```python
from build123d import *

# Parameters (mm, degrees)
SKETCH1_R           = 17.78
BOSS_EXTRUDE1_DEPTH = 1.5875
CUT_EXTRUDE1_DEPTH  = 2.5875


with BuildPart() as part:
    # Sketch1 → Boss-Extrude1 (new body)
    with BuildSketch(Plane(origin=(0, 0, 0), x_dir=(1, 0, 0), z_dir=(0, 1, 0))):
        Circle(SKETCH1_R)
    extrude(amount=BOSS_EXTRUDE1_DEPTH)

    # Sketch2 → Cut-Extrude1 (cut, through all)
    with BuildSketch(Plane(origin=(0, 1.5875, 0), x_dir=(1, 0, 0), z_dir=(0, 1, 0))):
        with BuildLine():
            Line((-0.670254455, 13.953911959), (-0.775316452, 12.67631194))
            ThreePointArc((-0.775316452, 12.67631194), (-1.327511483, 12.630428071), (-1.877179521, 12.560501465))
            Line((-1.877179521, 12.560501465), (-2.245573641, 13.788339241))
            ThreePointArc((-2.245573641, 13.788339241), (-2.904526321, 13.664721982), (-3.556789216, 13.509631767))
            Line((-3.556789216, 13.509631767), (-3.393927376, 12.238106756))
            ThreePointArc((-3.393927376, 12.238106756), (-3.924515829, 12.078417757), (-4.447633742, 11.895736803))
            Line((-4.447633742, 11.895736803), (-5.063259395, 13.020149934))
            ThreePointArc((-5.063259395, 13.020149934), (-5.682110904, 12.762230043), (-6.287875221, 12.474915839))
            Line((-6.287875221, 12.474915839), (-5.864207388, 11.265037581))
            ThreePointArc((-5.864207388, 11.265037581), (-6.35, 10.998522628), (-6.823705026, 10.711071362))
            Line((-6.823705026, 10.711071362), (-7.659656416, 11.682917597))
            ThreePointArc((-7.659656416, 11.682917597), (-8.211359975, 11.301967411), (-8.744150906, 10.894986229))
            Line((-8.744150906, 10.894986229), (-8.078193398, 9.799632209))
            ThreePointArc((-8.078193398, 9.799632209), (-8.497958701, 9.437939284), (-8.901547657, 9.058280704))
            Line((-8.901547657, 9.058280704), (-9.921289697, 9.835085701))
            ThreePointArc((-9.921289697, 9.835085701), (-10.381733212, 9.347754571), (-10.818265238, 8.83889344))
            Line((-10.818265238, 8.83889344), (-9.939123592, 7.905935885))
            ThreePointArc((-9.939123592, 7.905935885), (-10.274515829, 7.464872704), (-10.59034994, 7.009599713))
            Line((-10.59034994, 7.009599713), (-11.749315011, 7.557413365))
            ThreePointArc((-11.749315011, 7.557413365), (-12.098374891, 6.985), (-12.419569467, 6.396498594))
            Line((-12.419569467, 6.396498594), (-11.365666392, 5.666712226))
            ThreePointArc((-11.365666392, 5.666712226), (-11.602027312, 5.165555367), (-11.816303113, 4.654565579))
            Line((-11.816303113, 4.654565579), (-13.063838879, 4.949445801))
            ThreePointArc((-13.063838879, 4.949445801), (-13.286259533, 4.316967411), (-13.478078914, 3.674546066))
            Line((-13.478078914, 3.674546066), (-12.295475033, 3.179826051))
            ThreePointArc((-12.295475033, 3.179826051), (-12.422474529, 2.640478473), (-12.52582714, 2.096104594))
            Line((-12.52582714, 2.096104594), (-13.807410301, 2.125163705))
            ThreePointArc((-13.807410301, 2.125163705), (-13.893470878, 1.460262632), (-13.947531638, 0.791998242))
            Line((-13.947531638, 0.791998242), (-12.687912414, 0.55396622))
            ThreePointArc((-12.687912414, 0.55396622), (-12.7, 0), (-12.687912414, -0.55396622))
            Line((-12.687912414, -0.55396622), (-13.947531638, -0.791998242))
            ThreePointArc((-13.947531638, -0.791998242), (-13.893470878, -1.460262632), (-13.807410301, -2.125163705))
            Line((-13.807410301, -2.125163705), (-12.52582714, -2.096104594))
            ThreePointArc((-12.52582714, -2.096104594), (-12.422474529, -2.640478473), (-12.295475033, -3.179826051))
            Line((-12.295475033, -3.179826051), (-13.478078914, -3.674546066))
            ThreePointArc((-13.478078914, -3.674546066), (-13.286259533, -4.316967411), (-13.063838879, -4.949445801))
            Line((-13.063838879, -4.949445801), (-11.816303113, -4.654565579))
            ThreePointArc((-11.816303113, -4.654565579), (-11.602027312, -5.165555367), (-11.365666392, -5.666712226))
            Line((-11.365666392, -5.666712226), (-12.419569467, -6.396498594))
            ThreePointArc((-12.419569467, -6.396498594), (-12.098374891, -6.985), (-11.749315011, -7.557413365))
            Line((-11.749315011, -7.557413365), (-10.59034994, -7.009599713))
            ThreePointArc((-10.59034994, -7.009599713), (-10.274515829, -7.464872704), (-9.939123592, -7.905935885))
            Line((-9.939123592, -7.905935885), (-10.818265238, -8.83889344))
            ThreePointArc((-10.818265238, -8.83889344), (-10.381733212, -9.347754571), (-9.921289697, -9.835085701))
            Line((-9.921289697, -9.835085701), (-8.901547657, -9.058280704))
            ThreePointArc((-8.901547657, -9.058280704), (-8.497958701, -9.437939284), (-8.078193398, -9.799632209))
            Line((-8.078193398, -9.799632209), (-8.744150906, -10.894986229))
            ThreePointArc((-8.744150906, -10.894986229), (-8.211359975, -11.301967411), (-7.659656416, -11.682917597))
            Line((-7.659656416, -11.682917597), (-6.823705026, -10.711071362))
            ThreePointArc((-6.823705026, -10.711071362), (-6.35, -10.998522628), (-5.864207388, -11.265037581))
            Line((-5.864207388, -11.265037581), (-6.287875221, -12.474915839))
            ThreePointArc((-6.287875221, -12.474915839), (-5.682110904, -12.762230043), (-5.063259395, -13.020149934))
            Line((-5.063259395, -13.020149934), (-4.447633742, -11.895736803))
            ThreePointArc((-4.447633742, -11.895736803), (-3.924515829, -12.078417757), (-3.393927376, -12.238106756))
            Line((-3.393927376, -12.238106756), (-3.556789216, -13.509631767))
            ThreePointArc((-3.556789216, -13.509631767), (-2.904526321, -13.664721982), (-2.245573641, -13.788339241))
            Line((-2.245573641, -13.788339241), (-1.877179521, -12.560501465))
            ThreePointArc((-1.877179521, -12.560501465), (-1.327511483, -12.630428071), (-0.775316452, -12.67631194))
            Line((-0.775316452, -12.67631194), (-0.670254455, -13.953911959))
            ThreePointArc((-0.670254455, -13.953911959), (0, -13.97), (0.670254455, -13.953911959))
            Line((0.670254455, -13.953911959), (0.775316452, -12.67631194))
            ThreePointArc((0.775316452, -12.67631194), (1.327511483, -12.630428071), (1.877179521, -12.560501465))
            Line((1.877179521, -12.560501465), (2.245573641, -13.788339241))
            ThreePointArc((2.245573641, -13.788339241), (2.904526321, -13.664721982), (3.556789216, -13.509631767))
            Line((3.556789216, -13.509631767), (3.393927376, -12.238106756))
            ThreePointArc((3.393927376, -12.238106756), (3.924515829, -12.078417757), (4.447633742, -11.895736803))
            Line((4.447633742, -11.895736803), (5.063259395, -13.020149934))
            ThreePointArc((5.063259395, -13.020149934), (5.682110904, -12.762230043), (6.287875221, -12.474915839))
            Line((6.287875221, -12.474915839), (5.864207388, -11.265037581))
            ThreePointArc((5.864207388, -11.265037581), (6.35, -10.998522628), (6.823705026, -10.711071362))
            Line((6.823705026, -10.711071362), (7.659656416, -11.682917597))
            ThreePointArc((7.659656416, -11.682917597), (8.211359975, -11.301967411), (8.744150906, -10.894986229))
            Line((8.744150906, -10.894986229), (8.078193398, -9.799632209))
            ThreePointArc((8.078193398, -9.799632209), (8.497958701, -9.437939284), (8.901547657, -9.058280704))
            Line((8.901547657, -9.058280704), (9.921289697, -9.835085701))
            ThreePointArc((9.921289697, -9.835085701), (10.381733212, -9.347754571), (10.818265238, -8.83889344))
            Line((10.818265238, -8.83889344), (9.939123592, -7.905935885))
            ThreePointArc((9.939123592, -7.905935885), (10.274515829, -7.464872704), (10.59034994, -7.009599713))
            Line((10.59034994, -7.009599713), (11.749315011, -7.557413365))
            ThreePointArc((11.749315011, -7.557413365), (12.098374891, -6.985), (12.419569467, -6.396498594))
            Line((12.419569467, -6.396498594), (11.365666392, -5.666712226))
            ThreePointArc((11.365666392, -5.666712226), (11.602027312, -5.165555367), (11.816303113, -4.654565579))
            Line((11.816303113, -4.654565579), (13.063838879, -4.949445801))
            ThreePointArc((13.063838879, -4.949445801), (13.286259533, -4.316967411), (13.478078914, -3.674546066))
            Line((13.478078914, -3.674546066), (12.295475033, -3.179826051))
            ThreePointArc((12.295475033, -3.179826051), (12.422474529, -2.640478473), (12.52582714, -2.096104594))
            Line((12.52582714, -2.096104594), (13.807410301, -2.125163705))
            ThreePointArc((13.807410301, -2.125163705), (13.893470878, -1.460262632), (13.947531638, -0.791998242))
            Line((13.947531638, -0.791998242), (12.687912414, -0.55396622))
            ThreePointArc((12.687912414, -0.55396622), (12.7, 0), (12.687912414, 0.55396622))
            Line((12.687912414, 0.55396622), (13.947531638, 0.791998242))
            ThreePointArc((13.947531638, 0.791998242), (13.893470878, 1.460262632), (13.807410301, 2.125163705))
            Line((13.807410301, 2.125163705), (12.52582714, 2.096104594))
            ThreePointArc((12.52582714, 2.096104594), (12.422474529, 2.640478473), (12.295475033, 3.179826051))
            Line((12.295475033, 3.179826051), (13.478078914, 3.674546066))
            ThreePointArc((13.478078914, 3.674546066), (13.286259533, 4.316967411), (13.063838879, 4.949445801))
            Line((13.063838879, 4.949445801), (11.816303113, 4.654565579))
            ThreePointArc((11.816303113, 4.654565579), (11.602027312, 5.165555367), (11.365666392, 5.666712226))
            Line((11.365666392, 5.666712226), (12.419569467, 6.396498594))
            ThreePointArc((12.419569467, 6.396498594), (12.098374891, 6.985), (11.749315011, 7.557413365))
            Line((11.749315011, 7.557413365), (10.59034994, 7.009599713))
            ThreePointArc((10.59034994, 7.009599713), (10.274515829, 7.464872704), (9.939123592, 7.905935885))
            Line((9.939123592, 7.905935885), (10.818265238, 8.83889344))
            ThreePointArc((10.818265238, 8.83889344), (10.381733212, 9.347754571), (9.921289697, 9.835085701))
            Line((9.921289697, 9.835085701), (8.901547657, 9.058280704))
            ThreePointArc((8.901547657, 9.058280704), (8.497958701, 9.437939284), (8.078193398, 9.799632209))
            Line((8.078193398, 9.799632209), (8.744150906, 10.894986229))
            ThreePointArc((8.744150906, 10.894986229), (8.211359975, 11.301967411), (7.659656416, 11.682917597))
            Line((7.659656416, 11.682917597), (6.823705026, 10.711071362))
            ThreePointArc((6.823705026, 10.711071362), (6.35, 10.998522628), (5.864207388, 11.265037581))
            Line((5.864207388, 11.265037581), (6.287875221, 12.474915839))
            ThreePointArc((6.287875221, 12.474915839), (5.682110904, 12.762230043), (5.063259395, 13.020149934))
            Line((5.063259395, 13.020149934), (4.447633742, 11.895736803))
            ThreePointArc((4.447633742, 11.895736803), (3.924515829, 12.078417757), (3.393927376, 12.238106756))
            Line((3.393927376, 12.238106756), (3.556789216, 13.509631767))
            ThreePointArc((3.556789216, 13.509631767), (2.904526321, 13.664721982), (2.245573641, 13.788339241))
            Line((2.245573641, 13.788339241), (1.877179521, 12.560501465))
            ThreePointArc((1.877179521, 12.560501465), (1.327511483, 12.630428071), (0.775316452, 12.67631194))
            Line((0.775316452, 12.67631194), (0.670254455, 13.953911959))
            ThreePointArc((0.670254455, 13.953911959), (0, 13.97), (-0.670254455, 13.953911959))
        make_face()
    extrude(amount=-CUT_EXTRUDE1_DEPTH, mode=Mode.SUBTRACT)


solid = part.part
```
CAD build for the part. Positions are in the model's coordinates, mm. Give positions to 0.01 mm unless a question says otherwise; leave off trailing zeros. Write each loop counter-clockwise with the first axis right and the second up, starting at its lowest first coordinate (ties: lowest second). Pieces come first, ordered by that corner, then holes. Notation, with made-up numbers: (87, 34) -> (135, 34) arc R15 cw to (135, 63) -> close; hole circle Ø5 at (46, -26.75). An arc over 180 degrees is marked (long way). Write each question's results on one line, items separated by ' | '.
1. Cut at C-C, the plane x = -15. Write the cut outline in (y, z), then the cut area to 3 significant figures.
Geometry check:
outline: (0, -9.55) -> (1.59, -9.55) -> (1.59, 9.55) -> (0, 9.55) -> close | area: 30.3 mm²
2. Cut at A-A, the plane z = 0. Write the cut outline in (x, y).
Geometry check:
outline: (-17.78, 0) -> (-12.7, 0) -> (-12.7, 1.59) -> (-17.78, 1.59) -> close; (12.7, 0) -> (17.78, 0) -> (17.78, 1.59) -> (12.7, 1.59) -> close
3. Wall check: probe 1 along X at (y, z) = (1.2, 7.5); probe 2 along X at (y, z) = (0.9, 11); probe 3 along X at (y, z) = (1.3, -0.5). Give the ranges that are in metal, low to high. Write a range as [from, to].
Geometry check:
probe 1: [-16.12, -11.79], [-11.63, -10.25], [10.25, 11.63], [11.79, 16.12] | probe 2: [-13.97, -8.61], [-7.07, -6.35], [6.35, 7.07], [8.61, 13.97] | probe 3: [-17.77, -12.69], [12.69, 17.77]
4. Cut at B-B, the plane x = 0. Write the cut outline in (y, z).
Geometry check:
outline: (0, -17.78) -> (1.59, -17.78) -> (1.59, -13.97) -> (0, -13.97) -> close; (0, 13.97) -> (1.59, 13.97) -> (1.59, 17.78) -> (0, 17.78) -> close
